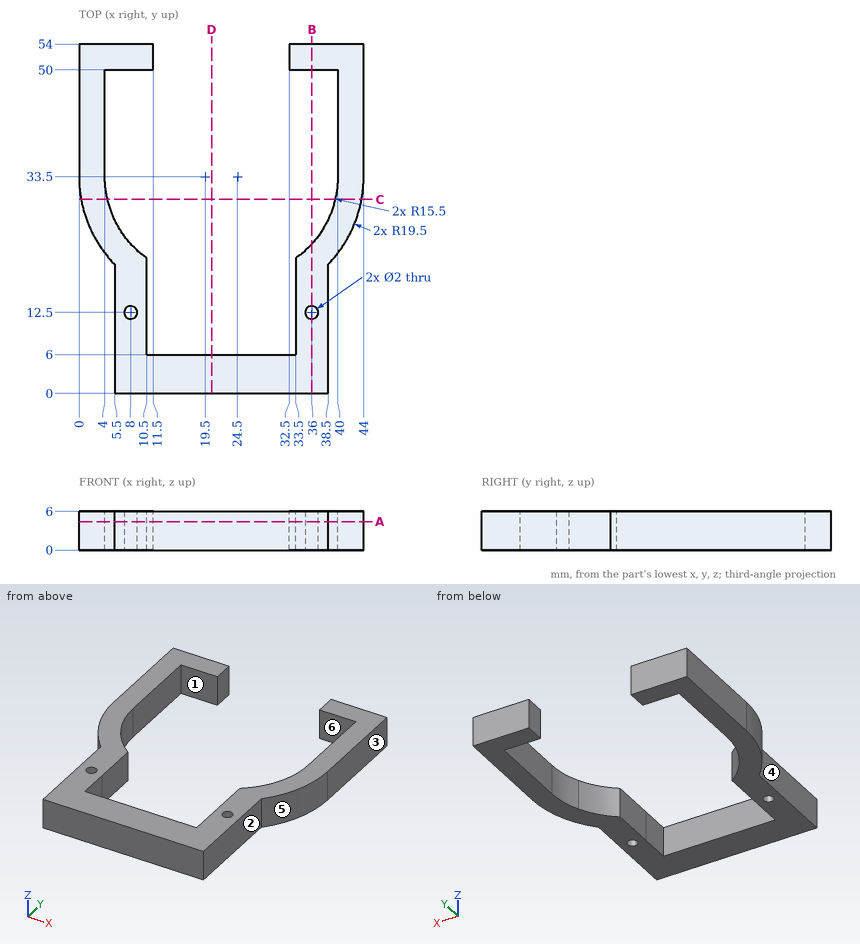
Study the drawing (mm; zero at the part's minimum x, y, z) and answer. A direction names the side the tool comes from. Coordinates: 2 decimals unless noted, no trailing zeros. Write each loop counter-clockwise with the first axis right and the second up, starting at its lowest first coordinate (ties: lowest second). Pieces come first, ordered by that corner, then holes. Notation, with made-up numbers: (28, -7) - (51, -7) arc R10 ccw to (51, 9) - close; hole circle Ø1 at (67.25, 66.5). An arc over 180 degrees is marked (long way). Answer as a JSON object with one key per item and string values. Group by question number.
1. Consider L1, parallel to X at y = 45.5, z = 0.9; L2, parallel to Y at x = 8, z = 1.9; L3, parallel to Y at x = 19.5, z = 5.5. Determine where each line is inside the solid, lowest interval first. Write a range as [from, to].
2. A cutting plane is placed at A-A (z = 4.4). Determine the outline of the cut face in (x, y), plus the area to 3 significant figures.
3. A cutting plane is placed at C-C (y = 30). Determine the outline of the cut face in (x, z), plus the area to 3 significant figures.
4. This flat-tipped pin is pushed along its axis until it touches: P1, Ø1.8, axis at y = 10.5, z = 4.5, coming from the -X side. Where does it stop, or does it pass through?
5. Which of the six approach directions +Z, -Z, +X, -X, +Y, -Y give full straight-line access (tool end or side, diameter ignored) to the marked faces 1, 2 and 3?
6. The mould has two halves that part along Y. Classify the marked faces 4, 5 and 6: +Y half, -Y half, draft (parallel to the pull), parting line (faces both ways), or undercut.
7. A cutting plane is placed at D-D (x = 20.5). Determine the outline of the cut face in (y, z).
8. A cutting plane is placed at B-B (x = 36). Determine the outline of the cut face in (y, z).
Worked out:
{
 "1": {"L1": "x = [0, 4], [40, 44]", "L2": "y = [0, 11.5], [13.5, 23.11], [50, 54]", "L3": "y = [0, 6]"},
 "2": {"outline": "(0, 33.5) arc R19.5 ccw to (5.5, 19.93) - (5.5, 0) - (38.5, 0) - (38.5, 19.93) arc R19.5 ccw to (44, 33.5) - (44, 54) - (32.5, 54) - (32.5, 50) - (40, 50) - (40, 33.5) arc R15.5 cw to (33.5, 20.88) - (33.5, 6) - (10.5, 6) - (10.5, 20.88) arc R15.5 cw to (4, 33.5) - (4, 50) - (11.5, 50) - (11.5, 54) - (0, 54) - close; hole circle Ø2 at (8, 12.5); hole circle Ø2 at (36, 12.5)", "area": "678 mm²"},
 "3": {"outline": "(0.32, 0) - (4.4, 0) - (4.4, 6) - (0.32, 6) - close; (39.6, 0) - (43.68, 0) - (43.68, 6) - (39.6, 6) - close", "area": "49.0 mm²"},
 "4": {"P1": "stops at x = 5.5"},
 "5": {"face 1": "+Z, -Z", "face 2": "+Z, -Z, +X, -Y", "face 3": "+Z, -Z, +X, +Y, -Y"},
 "6": {"face 4": "draft", "face 5": "-Y half", "face 6": "undercut"},
 "7": {"outline": "(0, 0) - (6, 0) - (6, 6) - (0, 6) - close"},
 "8": {"outline": "(0, 0) - (11.5, 0) - (11.5, 6) - (0, 6) - close; (13.5, 0) - (23.11, 0) - (23.11, 6) - (13.5, 6) - close; (50, 0) - (54, 0) - (54, 6) - (50, 6) - close"}
}
